Read the model definition and answer for the solid it produces. Units are mm, in the model's axes. Face numbers are marked on the shaded views. Coordinates: 2 decimals unless noted, no trailing zeros. Order: outer loops, then holes, each group sorted by start corner. A loop starts at its lowest first (then second) coordinate and runs counter-clockwise, first axis right, second up. Notation, with made-up numbers: (-21, -37.75) -> (18, -37.75) arc R25 ccw to (18, -17.75) -> close; hole circle Ø4 at (82, 3). An arc over 180 degrees is marked (long way). Answer in a Markdown table with one row per item.
from build123d import *

# Parameters (mm, degrees)
F0_R      = 27.5
F1_DEPTH  = 4
F2_R      = 24.75
F3_DEPTH  = 3
F4_R      = 22.5
F5_DEPTH  = 3
F6_R      = 20.5
F7_DEPTH  = 3
F8_R      = 18.5
F9_DEPTH  = 3
F10_R     = 16.5
F11_DEPTH = 3
F12_R     = 14.5
F13_DEPTH = 3
F14_R     = 12.5
F15_DEPTH = 3
F16_R     = 4
F17_DEPTH = 35
F18_SIZE  = 0.5
F19_SIZE  = 0.5


with BuildPart() as f1:
    # F0 (on Top) → F1 (new body)
    with BuildSketch(Plane.XY):
        Circle(F0_R)
    extrude(amount=F1_DEPTH)

    # F2 (on face) → F3 (join)
    with BuildSketch(Plane.XY.offset(4)):
        Circle(F2_R)
    extrude(amount=F3_DEPTH)

    # F4 (on face) → F5 (join)
    with BuildSketch(Plane.XY.offset(7)):
        Circle(F4_R)
    extrude(amount=F5_DEPTH)

    # F6 (on face) → F7 (join)
    with BuildSketch(Plane.XY.offset(10)):
        Circle(F6_R)
    extrude(amount=F7_DEPTH)

    # F8 (on face) → F9 (join)
    with BuildSketch(Plane.XY.offset(13)):
        Circle(F8_R)
    extrude(amount=F9_DEPTH)

    # F10 (on face) → F11 (join)
    with BuildSketch(Plane.XY.offset(16)):
        Circle(F10_R)
    extrude(amount=F11_DEPTH)

    # F12 (on face) → F13 (join)
    with BuildSketch(Plane.XY.offset(19)):
        Circle(F12_R)
    extrude(amount=F13_DEPTH)

    # F14 (on face) → F15 (join)
    with BuildSketch(Plane.XY.offset(22)):
        Circle(F14_R)
    extrude(amount=F15_DEPTH)

    # F16 (on face) → F17 (cut)
    with BuildSketch(Plane.XY.offset(25)):
        Circle(F16_R)
    extrude(amount=-F17_DEPTH, mode=Mode.SUBTRACT)

    # F18
    f18_edges = [f1.edges().sort_by_distance(p)[0] for p in [
        (-12.5, 0, 25),
    ]]
    chamfer(f18_edges, length=F18_SIZE)

    # F19
    f19_edges = [f1.edges().sort_by_distance(p)[0] for p in [
        (-14.5, 0, 22),
        (-16.5, 0, 19),
        (-18.5, 0, 16),
        (-20.5, 0, 13),
        (-22.5, 0, 10),
        (-24.75, 0, 7),
        (-27.5, 0, 4),
    ]]
    chamfer(f19_edges, length=F19_SIZE)


solid = f1.part
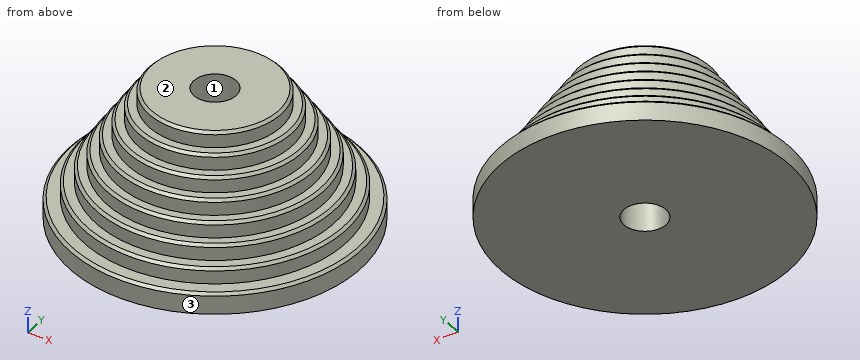
Q1. The part is cut by section A-A (z = 20). Write down the section's boundary in (x, y), then the cut area to 3 significant figures.
Outcome:
| item | result |
|---|---|
| outline | circle Ø29 at (0, 0); hole circle Ø8 at (0, 0) |
| area | 610 mm² |
Q2. For a pull along Y with two mould halves and no side action, classify the marked faces 1, 2 and 3 as pulls with the +Y half, pulls with the -Y half, needs draft (parallel to the pull), parting line crosses it, or undercut.
Outcome:
| item | result |
|---|---|
| face 1 | undercut |
| face 2 | needs draft |
| face 3 | parting line crosses it |
Q3. Consider line 1 (Y direction, x = 0, z = 17.25); line 2 (Z direction, x = 9.5, y = -17.5); line 3 (Y direction, x = 0, z = 9.25). Determine where each line is inside the solid, lowest interval first.
Outcome:
| item | result |
|---|---|
| line 1 | -16.5 to -4, 4 to 16.5 |
| line 2 | 0 to 13 |
| line 3 | -22.5 to -4, 4 to 22.5 |
Q4. Given pin 1 (1.5 mm diameter, centred on x = 0, z = 22, fed in from -Y); pin 2 (4 mm diameter, centred on x = 8.5, z = 3.5, fed in from +Y); pin 3 (2 mm diameter, centred on x = 3.5, z = 12, fed in from +Y), each flat-ended and moving along its own axis, determine where each tip first touches the part or whether it passes through.
Outcome:
| item | result |
|---|---|
| pin 1 | y = -14.5 |
| pin 2 | y = 26.72 |
| pin 3 | y = 20.35 |
